Read the model definition and answer for the solid it produces. Units are mm, in the model's axes. A direction names the side the tool comes from. Round coordinates to 2 decimals unless told otherwise and drop trailing zeros. Order: outer loops, then holes, each group sorted by start corner. A loop starts at its lowest first (then second) coordinate and runs counter-clockwise, first axis right, second up. Notation, with made-up numbers: (-21.5, -6.5) -> (19.5, -6.5) arc R18 ccw to (19.5, 5.5) -> close; hole circle Ø3 at (75.25, 37.25). An arc over 180 degrees is marked (long way). One line per item, written item: value. Start each with the question number.
1. Section D-D (x = 20) is taken. Give the vertices of the cut face in (y, z), then the cut area to 3 significant figures.
2. For faces 1 (the face through (41.99, 0.53, 4.93)), 2 (the face through (26.582, -13.897, 5.351)), 3 (the face through (0, 12.5, 5)), 4 (the face through (0, -12.5, 5)), 5 (the face through (-1, 0, 10)), determine the directions among +Z, -Z, +X, -X, +Y, -Y from which every point of the face is accessible in a straight line to the end or side of a thin tool.
3. Consider line 1 (Y direction, x = 0, z = 6); line 2 (X direction, y = -0.5, z = 7.75); line 3 (Z direction, x = -25, y = -14.25). Determine where each line is inside the solid, lowest interval first.
4. The mould has two halves that part along X. Classify faces 6 (the face through (-1, 0, 0)), 7 (the face through (-23.418, -13.897, 5.351)): released by +X, released by -X, zero draft, split by the parting line, or undercut.
5. Flat-ended cylindrical pins translate along their axes: pin 1 Ø3 at (x, z) = (15.5, 1.5) entering from +Y; pin 2 Ø3 at (y, z) = (10.5, 8.5) entering from +X; pin 3 Ø3 at (x, z) = (-31.5, 2.5) entering from +Y. Find the tip coordinate at first contact, or state that the pin passes through.
6. Section C-C (z = 7.75) is taken. Give the vertices of the cut face in (x, y), then the cut area to 3 significant figures.
7. Section A-A (x = 0) is taken. Give the vertices of the cut face in (y, z).
8. Section B-B (y = 0) is taken. Give the vertices of the cut face in (x, z).
Autodesk Inventor part; units mm, degrees
ref_plane "Arbeitsebene1" through (25, -17, 0) normal (0, 1, 0) x (-1, 0, 0)
ref_plane "YZ Plane" through (0, 0, 0) normal (1, 0, 0) x (0, 1, 0)
ref_plane "XY Plane" through (0, 0, 0) normal (0, 0, 1) x (1, 0, 0)
sketch "Skizze1" plane through (0, 0, 0) normal (0, 0, 1) x (1, 0, 0)
  line L0 (-58.8, 0) -> (58.8, 0)
  line L1 (0, -24.5) -> (0, 24.5)
  circle A0 centre (-25, 0) radius 11
  circle A1 centre (25, 0) radius 11
  arc A2 (-14.6978, 13.5227) -> (-14.6978, -13.5227) centre (-25, 0) ccw
  arc A3 (14.6978, -13.5227) -> (14.6978, 13.5227) centre (25, 0) ccw
  line L2 (11.6677, -12.5) -> (-11.6677, -12.5)
  line L3 (-11.6677, 12.5) -> (11.6677, 12.5)
  arc A4 (-11.6677, -12.5) -> (-14.6978, -13.5227) centre (-11.6677, -17.5) ccw
  arc A5 (14.6978, -13.5227) -> (11.6677, -12.5) centre (11.6677, -17.5) ccw
  arc A6 (11.6677, 12.5) -> (14.6978, 13.5227) centre (11.6677, 17.5) ccw
  arc A7 (-14.6978, 13.5227) -> (-11.6677, 12.5) centre (-11.6677, 17.5) ccw
  point P0 (0, 0)
  point P1 (-13.4783, -12.5)
  point P2 (13.4783, 12.5)
  point P3 (13.4783, -12.5)
  point P4 (-13.4783, 12.5)
  dimension "d0" = 50
  dimension "d1" = 22
  dimension "d2" = 34
  dimension "d4" = 25
  dimension "d5" = 5
  dimension "d6" = 6
extrude "Extrusion1" add sketch "Skizze1" along normal blind 10 contours A2 A7 L3 L1 L0 A0 | L0 A0 L1 L2 A4 A2 | L1 L3 A6 A3 L0 A1 | L0 A1 A3 A5 L2 L1
ref_plane "Arbeitsebene1" through (25, -17, 0) normal (0, 1, 0) x (-1, 0, 0)
sketch "Skizze2" plane through (25, -17, 0) normal (0, 1, 0) x (-1, 0, 0)
  line L0 (-33.8, 0) -> (83.8, 0)
  line L1 (25, -2) -> (25, 12)
  line L2 (39.6978, 10) -> (67, 10)
  line L3 (-17, 10) -> (10.3022, 10)
  line L4 (-17, 0) -> (-17, 10)
  line L5 (67, 0) -> (67, 10)
  line L6 (67, 5) -> (-17, 5)
  point P0 (25, 0)
  point P1 (50, 5)
  point P2 (0, 5)
  dimension "d9" = 50
hole "Bohrung1" at (-25, -17, 5) at (25, -17, 5) direction (0, 1, 0) diameter 3.242 depth 8 tip angle 118
sketch "Skizze3" plane through (0, 0, 10) normal (0, 0, 1) x (1, 0, 0)
  circle A0 centre (0, -8) radius 1.5
  circle A1 centre (0, 8) radius 1.5
  point P0 (0, 0)
hole "Bohrung2" at (0, 8, 10) at (0, -8, 10) direction (0, 0, -1) diameter 5 end through all
properties part number "13_0204_047"
Answer:
1. outline: (-16.25, 0) -> (-9.8, 0) -> (-9.8, 10) -> (-16.25, 10) -> close; (9.8, 0) -> (16.25, 0) -> (16.25, 10) -> (9.8, 10) -> close
1. area: 129 mm^2
2. face 1: +Z, -Z
2. face 2: -Y
2. face 3: +Z, -Z, +Y
2. face 4: +Z, -Z, -Y
2. face 5: +Z, +X, -X, +Y, -Y
3. line 1: -12.5 to -10.5, -5.5 to 5.5, 10.5 to 12.5
3. line 2: -41.99 to -35.99, -14.01 to 14.01, 35.99 to 41.99
3. line 3: 0 to 3.38, 6.62 to 10
4. face 6: zero draft
4. face 7: undercut
5. pin 1: y = 15
5. pin 2: x = 39.42
5. pin 3: y = 16.25
6. outline: (-14.7, -13.52) arc R5 cw to (-11.67, -12.5) -> (11.67, -12.5) arc R5 cw to (14.7, -13.52) arc R17 ccw (long way) to (14.7, 13.52) arc R5 cw to (11.67, 12.5) -> (-11.67, 12.5) arc R5 cw to (-14.7, 13.52) arc R17 ccw (long way) to start; hole circle Ø22 at (-25, 0); hole circle Ø5 at (0, -8); hole circle Ø5 at (0, 8); hole circle Ø22 at (25, 0)
6. area: 1,500 mm^2
7. outline: (-12.5, 0) -> (-10.5, 0) -> (-10.5, 10) -> (-12.5, 10) -> close; (-5.5, 0) -> (5.5, 0) -> (5.5, 10) -> (-5.5, 10) -> close; (10.5, 0) -> (12.5, 0) -> (12.5, 10) -> (10.5, 10) -> close
8. outline: (-42, 0) -> (-36, 0) -> (-36, 10) -> (-42, 10) -> close; (-14, 0) -> (14, 0) -> (14, 10) -> (-14, 10) -> close; (36, 0) -> (42, 0) -> (42, 10) -> (36, 10) -> close
